from build123d import *

# Parameters (mm, degrees)
SKETCH1_R             = 60.625
SKETCH1_R_2           = 45
BOSS_EXTRUDE1_DEPTH   = 4
SKETCH2_R             = 49
SKETCH2_R_2           = 45
BOSS_EXTRUDE2_DEPTH   = 50.5
SKETCH4_W             = 8
SKETCH4_H             = 40.5
BOSS_EXTRUDE4_DEPTH   = 7
SKETCH4_W_2           = 27
SKETCH4_H_2           = 10
BOSS_EXTRUDE4_2_DEPTH = 7
BOSS_EXTRUDE5_DEPTH   = 4
SKETCH6_R             = 5
CUT_EXTRUDE2_DEPTH    = 52
CUT_EXTRUDE6_DEPTH    = 100.503925853
BOSS_EXTRUDE6_DEPTH   = 6.75


with BuildPart() as part:
    # Sketch1 → Boss-Extrude1 (new body)
    with BuildSketch(Plane(origin=(0, 0, 0), x_dir=(1, 0, 0), z_dir=(0, 1, 0))):
        with Locations(Location((0, 0, 0), (0, 0, 270))):
            Circle(SKETCH1_R)
        with Locations(Location((0, 0, 0), (0, 0, 270))):
            Circle(SKETCH1_R_2, mode=Mode.SUBTRACT)
    extrude(amount=BOSS_EXTRUDE1_DEPTH)

    # Sketch2 → Boss-Extrude2 (add)
    with BuildSketch(Plane(origin=(0, 4, 0), x_dir=(1, 0, 0), z_dir=(0, 1, 0))):
        with Locations(Location((0, 0, 0), (0, 0, 270))):
            Circle(SKETCH2_R)
        with Locations(Location((0, 0, 0), (0, 0, 270))):
            Circle(SKETCH2_R_2, mode=Mode.SUBTRACT)
    extrude(amount=BOSS_EXTRUDE2_DEPTH)



with BuildPart() as body_2:
    # Sketch4 → Boss-Extrude4 (new, symmetric)
    with BuildSketch(Plane.XY):
        with Locations((10, 20.25)):
            Rectangle(SKETCH4_W, SKETCH4_H)
    extrude(amount=BOSS_EXTRUDE4_DEPTH, both=True)


with BuildPart() as body_3:
    # Sketch4 → Boss-Extrude4 2 (new, symmetric)
    with BuildSketch(Plane.XY):
        with Locations((-30.5, 35.5)):
            Rectangle(SKETCH4_W_2, SKETCH4_H_2)
    extrude(amount=BOSS_EXTRUDE4_2_DEPTH, both=True)


with BuildPart() as part_1:
    add(part.part)

    add(body_2.part)  # Boss-Extrude5 merges body 2
    # Sketch5 → Boss-Extrude5 (add)
    with BuildSketch(Plane(origin=(0, 0, 0.832419338), x_dir=(1, 0, 0), z_dir=(0, -1, 0))):
        with BuildLine():
            Line((0.92268666, 14.579552818), (36.10584122, 30.137929754))
            ThreePointArc((36.10584122, 30.137929754), (47.46850162, -1.287411864), (36.651216878, -32.904630242))
            Line((36.651216878, -32.904630242), (0.92268666, -16.029114558))
            Line((0.92268666, -16.029114558), (0.92268666, 14.579552818))
        make_face()
    extrude(amount=-BOSS_EXTRUDE5_DEPTH)

    # Sketch6 → Cut-Extrude2 (cut)
    with BuildSketch(Plane.XY):
        with Locations(Location((-11.847358964, 24.485616242, 0), (0, 0, 180))):
            Circle(SKETCH6_R)
    extrude(amount=CUT_EXTRUDE2_DEPTH, mode=Mode.SUBTRACT)

    # Sketch11 → Cut-Extrude6 (cut, through all)
    with BuildSketch(Plane(origin=(0, 4, 0), x_dir=(1, 0, 0), z_dir=(0, 1, 0))):
        with BuildLine():
            Line((16.265526008, 12.732401326), (16.265526008, -6.549664017))
            Line((16.265526008, -6.549664017), (5.714961953, -6.549664017))
            Line((5.714961953, -6.549664017), (5.714961953, -11.643039768))
            Line((5.714961953, -11.643039768), (30.818028154, -22.557416377))
            ThreePointArc((30.818028154, -22.557416377), (39.374347706, -1.214976289), (32.152007517, 20.615006655))
            Line((32.152007517, 20.615006655), (16.265526008, 12.732401326))
        make_face()
    extrude(amount=-CUT_EXTRUDE6_DEPTH, mode=Mode.SUBTRACT)


    add(body_3.part)  # Boss-Extrude6 merges body 3
    # Sketch17 → Boss-Extrude6 (add, symmetric)
    with BuildSketch(Plane.XY):
        Polygon((-17, 30.5), (-45, 30.5), (-45, 12.445827276), (-18.590132897, 25.433454532), align=None)
    extrude(amount=BOSS_EXTRUDE6_DEPTH, both=True)


solid = part_1.part
Work out the finished part from the listing and answer in its coordinate system (mm). A direction names the side the tool comes from. Coordinates: 2 decimals unless noted, no trailing zeros. Loops run counter-clockwise (first coordinate to the right, second up) from the corner with the lowest first, then second, coordinate; pieces in that order, holes last. Notation, with made-up numbers: M 53.5,66.5 L 84.5,66.5 A22 ccw 84.5,96.5 Z; hole C 69.25,-8.75 d1. An arc over 180 degrees is marked long. Answer in a Markdown table with one row per item. Add a question column.
1. Flat-ended cylindrical pins translate along their axes: P1, Ø5, axis at x = -40.5, y = 47.5, coming from the +Z side; P2, Ø8, axis at x = 44, y = 6, coming from the +Z side; P3, Ø10, axis at x = -27.5, y = 39, coming from the -Z side. Find the tip coordinate at first contact, or state that the pin passes through.
2. Find section D-D, the plane z = 35.5. Write down the section's boundary in (x, y) (3 decimals).
3. Find section C-C, the plane x = -29. Write down the section's boundary in (y, z).
4. Consider L1, parallel to X at y = 9, z = -1.5 (3 decimals); L2, parallel to Z at x = 1, y = 19; L3, parallel to X at y = 43, z = 0. Determine where each line is inside the solid, lowest interval first.
5. Find section A-A, the plane y = 10. Write down the section's boundary in (x, z), then the cut area to 3 significant figures.
6. The mould has two halves that part along X. Classify faces 1 (the flat face through (11, 2, 6.55)), 2 (the flat face through (-49, 4, -5)), 3 (the cylindrical face through (-36.9, 2, -48.1)): pulls with the +X half, pulls with the -X half, needs draft (parallel to the pull), parting line crosses it, or undercut.
7. Find section B-B, the plane z = 20. Write down the section's boundary in (x, y), then the cut area to 3 significant figures.
8. A tool of negligible diameter and unlimited length cuts with its end or side. For faces 4 (the flat face through (10, 40.5, 0)), 5 (the flat face through (-31.98, 18.85, 0.09)), 6 (the flat face through (-22, 54.5, 40)), 7 (the flat face through (16.266, 2, -3)), from which of +Z, -Z, +X, -X, +Y, -Y can it reach the whole face along a straight path? Write none if from no direction.
Reported:
| question | item | result |
|---|---|---|
| 1 | P1 | stops at z = 30.94 |
| 1 | P2 | stops at z = 45.08 |
| 1 | P3 | stops at z = -43.53 |
| 2 | outline | M -49.144,0 L -27.654,0 L -27.654,54.5 L -33.775,54.5 L -33.775,4 L -49.144,4 Z; M 27.654,0 L 49.144,0 L 49.144,4 L 33.775,4 L 33.775,54.5 L 27.654,54.5 Z |
| 3 | outline | M 0,-53.24 L 4,-53.24 L 4,-39.5 L 54.5,-39.5 L 54.5,-34.41 L 0,-34.41 Z; M 0,34.41 L 54.5,34.41 L 54.5,39.5 L 4,39.5 L 4,53.24 L 0,53.24 Z; M 20.31,-6.75 L 30.5,-6.75 L 30.5,-7 L 40.5,-7 L 40.5,7 L 30.5,7 L 30.5,6.75 L 20.31,6.75 Z |
| 4 | L1 | x = -48.977 to -44.975, 6 to 14, 44.975 to 48.977 |
| 4 | L2 | z = -48.99 to -44.99, 44.99 to 48.99 |
| 4 | L3 | x = -49 to -45, 45 to 49 |
| 5 | outline | C 0,0 d98; M 6,-7 L 14,-7 L 14,7 L 6,7 Z; hole C 0,0 d90 |
| 5 | area | 1,290 mm^2 |
| 6 | face 1 | undercut |
| 6 | face 2 | needs draft |
| 6 | face 3 | parting line crosses it |
| 7 | outline | M -57.23,0 L -40.31,0 L -40.31,54.5 L -44.73,54.5 L -44.73,4 L -57.23,4 Z; M 11.3,0 L 24.94,0 L 24.94,4 L 11.3,4 Z; M 32.9,0 L 57.23,0 L 57.23,4 L 44.73,4 L 44.73,54.5 L 40.31,54.5 L 40.31,4 L 32.9,4 Z |
| 7 | area | 666 mm^2 |
| 8 | face 4 | +Y |
| 8 | face 5 | -Y |
| 8 | face 6 | +Z, -Z, +X, -X, +Y |
| 8 | face 7 | +Y, -Y |
